For this review, take the finished solid that the model builds, in its own axes (mm). A direction names the side the tool comes from. Coordinates: 2 decimals unless noted, no trailing zeros. Loops run counter-clockwise (first coordinate to the right, second up) from the corner with the lowest first, then second, coordinate; pieces in that order, holes last. Notation, with made-up numbers: (37, 54) -> (76, 54) arc R28 ccw to (76, 89) -> close; hole circle Ø2 at (31, 57). An arc over 180 degrees is marked (long way). Answer in a Markdown table with one row per item.
Autodesk Inventor part; units mm, degrees
ref_plane "YZ Plane" through (0, 0, 0) normal (1, 0, 0) x (0, 1, 0)
ref_plane "XZ Plane" through (0, 0, 0) normal (0, 1, 0) x (-1, 0, 0)
ref_plane "XY Plane" through (0, 0, 0) normal (0, 0, 1) x (1, 0, 0)
sketch "Эскиз1" plane through (0, 0, 0) normal (0, 0, 1) x (1, 0, 0)
  line L0 (0, 45) -> (0, -45)
  line L1 (0, -45) -> (13, -45)
  line L2 (14, -44) -> (14, -41)
  line L3 (14, -41) -> (10, -41)
  line L4 (9, -40) -> (9, -8.5)
  line L5 (8.5, -8) -> (7, -8)
  line L6 (6, -7) -> (6, 44)
  line L7 (5, 45) -> (0, 45)
  line L8 (14, -44) -> (13, -45)
  arc A0 (9, -40) -> (10, -41) centre (10, -40) ccw
  line L9 (9, -8.5) -> (8.5, -8)
  arc A1 (6, -7) -> (7, -8) centre (7, -7) ccw
  line L10 (6, 44) -> (5, 45)
  point P0 (0, 0)
  point P1 (0, 0)
  point P2 (14, -45)
  point P3 (9, -8)
  point P4 (6, 45)
  dimension "d0" = 90
  dimension "d1" = 28
  dimension "d2" = 1
  dimension "d3" = 45
  dimension "d4" = 4
  dimension "d5" = 1
  dimension "d6" = 18
  dimension "d7" = 0.5
  dimension "d8" = 45
  dimension "d9" = 1
  dimension "d10" = 12
  dimension "d11" = 33
  dimension "d12" = 1
  dimension "d13" = 45
revolve "Вращение1" add sketch "Эскиз1" angle 360 about axis through (0, 45, 0) along (0, -1, 0)
sketch "Эскиз2" plane through (0, -45, 0) normal (0, -1, 0) x (1, 0, 0)
  line L0 (0, 11) -> (0, -11) construction
  line L1 (-14, 14) -> (14, 14)
  line L2 (14, 14) -> (14, 11)
  line L3 (14, 11) -> (-14, 11)
  line L4 (-14, 11) -> (-14, 14)
  circle A0 centre (0, 0) radius 14
  point P0 (0, 0)
  point P1 (0, 0)
  dimension "d15" = 22
  dimension "d16" = 28
extrude "Выдавливание1" cut sketch "Эскиз2" against normal through all contours L1 A0 L3 L4 | L1 L2 L3 A0 | A0 L3 picked at (2.0072, 11.5463)
mirror "Зеркальное отражение1" about plane through (0, 0, 0) normal (0, 0, 1) of "Выдавливание1"
thread "Резьба1"
properties part number "62. Ось рычага управления"
Item 1: Take a section at A-A, the plane z = 0. State the section outline as (x, y) points.
Worked answers:
| item | result |
|---|---|
| outline | (-14, -44) -> (-13, -45) -> (13, -45) -> (14, -44) -> (14, -41) -> (10, -41) arc R1 cw to (9, -40) -> (9, -8.5) -> (8.5, -8) -> (7, -8) arc R1 cw to (6, -7) -> (6, 44) -> (5, 45) -> (-5, 45) -> (-6, 44) -> (-6, -7) arc R1 cw to (-7, -8) -> (-8.5, -8) -> (-9, -8.5) -> (-9, -40) arc R1 cw to (-10, -41) -> (-14, -41) -> close |
Item 2: For faces 1 (the cylindrical face through (-6, 19, 0)), 2 (the flat face through (0, 45, 0)), list the 3-axis set-ups (+Z, -Z, +X, -X, +Y, -Y) from which the entire face can be reached by the end or side of a thin tool; tool diameter is ignored.
Worked answers:
| item | result |
|---|---|
| face 1 | +Y |
| face 2 | +Z, -Z, +X, -X, +Y |
Item 3: Take a section at C-C, the plane y = 10. State the section outline as (x, z) points, and give its area (3 significant figures).
Worked answers:
| item | result |
|---|---|
| outline | circle Ø12 at (0, 0) |
| area | 113 mm² |
Item 4: Take a section at D-D, the plane y = -21. State the section outline as (x, z) points, and give its area (3 significant figures).
Worked answers:
| item | result |
|---|---|
| outline | circle Ø18 at (0, 0) |
| area | 254 mm² |
Item 5: Insertion check: pin 1 (3 mm diameter, centred on x = 2.5, y = 7, fed in from +Z); pin 2 (5 mm diameter, centred on y = 11.5, z = -7, fed in from +X); pin 3 (2 mm diameter, centred on y = 13, z = -2.5, fed in from +X). Each pin has a flat end and moves straight along its axis. Give the tip position at first contact, or say it passes through.
Worked answers:
| item | result |
|---|---|
| pin 1 | z = 5.92 |
| pin 2 | x = 3.97 |
| pin 3 | x = 5.81 |
Item 6: Take a section at B-B, the plane x = 0. State the section outline as (y, z) points, and give its area (3 significant figures).
Worked answers:
| item | result |
|---|---|
| outline | (-45, -11) -> (-41, -11) -> (-41, -10) arc R1 cw to (-40, -9) -> (-8.5, -9) -> (-8, -8.5) -> (-8, -7) arc R1 cw to (-7, -6) -> (44, -6) -> (45, -5) -> (45, 5) -> (44, 6) -> (-7, 6) arc R1 cw to (-8, 7) -> (-8, 8.5) -> (-8.5, 9) -> (-40, 9) arc R1 cw to (-41, 10) -> (-41, 11) -> (-45, 11) -> close |
| area | 1,320 mm² |
Item 7: For L1, parallel to Y at x = 10.5, z = -4.25; L2, parallel to X at y = -37, z = 3; L3, parallel to Y at x = 7.25, z = 0.5, list the stretches that pass through material, from the lowest coordinate up.
Worked answers:
| item | result |
|---|---|
| L1 | -45 to -41 |
| L2 | -8.49 to 8.49 |
| L3 | -45 to -8 |
